Here's how the part is built. I have some questions about the finished solid (model axes, mm). A direction names the side the tool comes from. Give positions to 0.01 mm unless a question says otherwise; leave off trailing zeros. Loops run counter-clockwise (first coordinate to the right, second up) from the corner with the lowest first, then second, coordinate; pieces in that order, holes last. Notation, with made-up numbers: (63, 41) - (115, 41) arc R22 cw to (115, 53) - close; hole circle Ø9 at (4.5, -32.75). An arc over 180 degrees is marked (long way). Return JSON: item names as keys, results as strings. Group by question number.
(1) For P1, Ø12, axis at x = -69.5, y = 18, coming from the -Z side, with a flat end and sliding along its axis, tell me the tip position at first contact or that it passes through.
(2) If we section it at A-A (z = -6.75): Please give me the cut outline in (x, y), then the cut area to 3 significant figures.
(3) If we section it at C-C (x = 76): Please give me the cut outline in (y, z).
(4) On a 3-axis mill with a long thin cutter (end or side, diameter ignored), from which of +Z, -Z, +X, -X, +Y, -Y can I reach the whole of each face in a straight line? I mean faces 4 (the flat face through (-4, 0, 2.54)), 5 (the flat face through (-4, -35.56, -8)). Say none if no direction works.
(5) If we section it at B-B (y = 26): Please give me the cut outline in (x, z).
(6) If we mould it in two halves opening along X, with no side actions, what happens to faces 1 (the flat face through (304.8, -1, -8)), 2 (the flat face through (-302.26, 0, -8)), 3 (the flat face through (-4, -38.1, -8))? For each: released by +X, released by -X, zero draft, split by the parting line, or undercut.
(7) I need wall thicknesses on probe 1 along Y at (x, z) = (-30, -4.25); probe 2 along X at (y, z) = (24, -6.5); probe 3 along Z at (x, y) = (-151, -10). Which ranges of each line are inside material? Lowest first, please. Write a range as [from, to].
```python
from build123d import *

# Parameters (mm, degrees)
SKETCH1_W           = 609.6
SKETCH1_H           = 76.2
BOSS_EXTRUDE1_DEPTH = 2.54
SKETCH2_W           = 609.6
SKETCH2_H           = 76.2
SKETCH2_W_2         = 604.52
SKETCH2_H_2         = 71.12
BOSS_EXTRUDE2_DEPTH = 19.05
FILLET1_R           = 2.54


with BuildPart() as part:
    # Sketch1 → Boss-Extrude1 (new body)
    with BuildSketch(Plane.XY):
        Rectangle(SKETCH1_W, SKETCH1_H)
    extrude(amount=BOSS_EXTRUDE1_DEPTH)

    # Sketch2 → Boss-Extrude2 (add)
    with BuildSketch(Plane.XY.offset(2.54)):
        Rectangle(SKETCH2_W, SKETCH2_H)
        Rectangle(SKETCH2_W_2, SKETCH2_H_2, mode=Mode.SUBTRACT)
    extrude(amount=-BOSS_EXTRUDE2_DEPTH)

    # Fillet1
    fillet1_edges = [part.edges().sort_by_distance(p)[0] for p in [
        (-304.8, 0, 2.54),
        (0, -38.1, 2.54),
        (304.8, 0, 2.54),
        (0, 38.1, 2.54),
    ]]
    fillet(fillet1_edges, radius=FILLET1_R)


solid = part.part
```
Values:
{
 "1": {"P1": "z = 0"},
 "2": {"outline": "(-304.8, -38.1) - (304.8, -38.1) - (304.8, 38.1) - (-304.8, 38.1) - close; hole (-302.26, -35.56) - (302.26, -35.56) - (302.26, 35.56) - (-302.26, 35.56) - close", "area": "3,460 mm2"},
 "3": {"outline": "(-38.1, -16.51) - (-35.56, -16.51) - (-35.56, 0) - (35.56, 0) - (35.56, -16.51) - (38.1, -16.51) - (38.1, 0) arc R2.54 ccw to (35.56, 2.54) - (-35.56, 2.54) arc R2.54 ccw to (-38.1, 0) - close"},
 "4": {"face 4": "+Z, +X, -X, +Y, -Y", "face 5": "-Z"},
 "5": {"outline": "(-304.8, -16.51) - (-302.26, -16.51) - (-302.26, 0) - (302.26, 0) - (302.26, -16.51) - (304.8, -16.51) - (304.8, 0) arc R2.54 ccw to (302.26, 2.54) - (-302.26, 2.54) arc R2.54 ccw to (-304.8, 0) - close"},
 "6": {"face 1": "released by +X", "face 2": "undercut", "face 3": "zero draft"},
 "7": {"probe 1": "[-38.1, -35.56], [35.56, 38.1]", "probe 2": "[-304.8, -302.26], [302.26, 304.8]", "probe 3": "[0, 2.54]"}
}
